from build123d import *

# Parameters (mm, degrees)
SKETCH1_R          = 10.5
EXTRUDE1_DEPTH     = 40
SKETCH2_R          = 2.5
EXTRUDE2_DEPTH     = 22.5
SKETCH3_R          = 13
SKETCH3_R_2        = 10.5
EXTRUDE3_DEPTH     = 3
SKETCH4_R          = 1.5
CUT_EXTRUDE1_DEPTH = 14
SKETCH7_R          = 2.2
CUT_EXTRUDE2_DEPTH = 1.5
CUT_EXTRUDE2_DRAFT = -26
SKETCH8_R          = 2.2
CUT_EXTRUDE3_DEPTH = 1.5
CUT_EXTRUDE3_TAPER = 26


with BuildPart() as part:
    # Sketch1 → Extrude1 (new body)
    with BuildSketch(Plane(origin=(0, 0, 0), x_dir=(1, 0, 0), z_dir=(0, 1, 0))):
        with Locations(Location((0, 0, 0), (0, 0, 270))):
            Circle(SKETCH1_R)
    extrude(amount=EXTRUDE1_DEPTH)

    # Sketch2 → Extrude2 (cut)
    with BuildSketch(Plane.XZ):
        with Locations(Location((0, 0, 0), (0, 0, 270))):
            Circle(SKETCH2_R)
    extrude(amount=-EXTRUDE2_DEPTH, mode=Mode.SUBTRACT)

    # Sketch3 → Extrude3 (add)
    with BuildSketch(Plane.XZ.offset(-6)):
        with Locations(Location((0, 0, 0), (0, 0, 270))):
            Circle(SKETCH3_R)
        with Locations(Location((0, 0, 0), (0, 0, 270))):
            Circle(SKETCH3_R_2, mode=Mode.SUBTRACT)
    extrude(amount=-EXTRUDE3_DEPTH)

    # Sketch4 → Cut-Extrude1 (cut, symmetric)
    with BuildSketch(Plane.XY):
        with Locations((0, 15.131749204)):
            Circle(SKETCH4_R)
    extrude(amount=CUT_EXTRUDE1_DEPTH, both=True, mode=Mode.SUBTRACT)


with BuildPart() as cut_extrude2_tool:
    # Sketch7 → Cut-Extrude2 (with draft: the straight prism first)
    with BuildSketch(Plane(origin=(0, 24.5, 10.5), x_dir=(-1, 0, 0), z_dir=(0, 0, 1))):
        with Locations((0, 9.368250796)):
            Circle(SKETCH7_R)
    extrude(amount=-CUT_EXTRUDE2_DEPTH)
    # Cut-Extrude2: the draft: its side faces are tilted about the plane it starts from
    cut_extrude2_sides = [cut_extrude2_tool.faces().sort_by_distance(p)[0] for p in [
        (2.2, 15.131749204, 9.75),
    ]]
    draft(cut_extrude2_sides, Plane(origin=(0, 24.5, 10.5), x_dir=(-1, 0, 0), z_dir=(0, 0, 1)), CUT_EXTRUDE2_DRAFT)


with BuildPart() as part_1:
    add(part.part)

    # Cut-Extrude2: cut by cut_extrude2_tool
    add(cut_extrude2_tool.part, mode=Mode.SUBTRACT)

    # Sketch8 → Cut-Extrude3 (cut)
    with BuildSketch(Plane.XY.offset(-10.5)):
        with Locations((0, 15.131749204)):
            Circle(SKETCH8_R)
    extrude(amount=CUT_EXTRUDE3_DEPTH, taper=CUT_EXTRUDE3_TAPER, mode=Mode.SUBTRACT)


solid = part_1.part
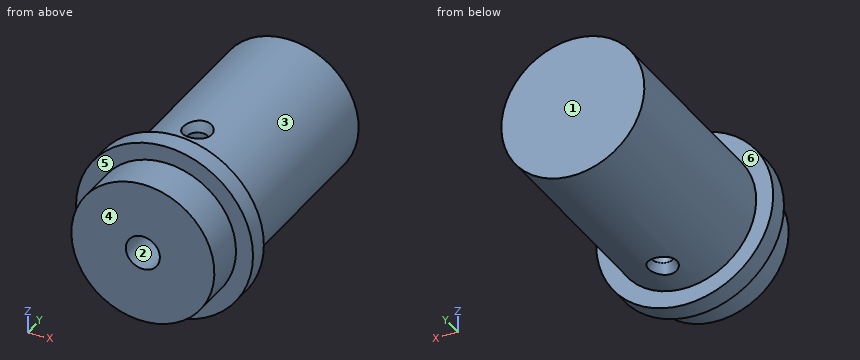
Read the model definition and answer for the solid it produces. Units are mm, in the model's axes. Face numbers are marked on the shaded views. A direction names the side the tool comes from. Round coordinates to 2 decimals unless told otherwise and drop trailing zeros. Order: outer loops, then holes, each group sorted by start corner. A loop starts at its lowest first (then second) coordinate and runs counter-clockwise, first axis right, second up.
1) The part is cut by section A-A on x = 0. Write down the section's boundary in (y, z), plus the area to 3 significant figures.
2) The part is cut by section C-C on z = 6.75. Write down the section's boundary in (x, y), plus the area to 3 significant figures.
3) The mould has two halves that part along X. Classify the marked faces 1, 2 and 3: released by +X, released by -X, zero draft, split by the parting line, or undercut.
4) For the marked faces 4, 5 and 6, determine the directions among +Z, -Z, +X, -X, +Y, -Y from which every point of the face is accessible in a straight line to the end or side of a thin tool.
5) Straight lines are drawn through the part: L1, parallel to Y at x = 0, z = 5.75; L2, parallel to Y at x = -1.5, z = -11.25; L3, parallel to Y at x = 0.25, z = -4.5. For each, find the intervals that lie inside material, in ascending order.
6) The part is cut by section D-D on x = 7.75. Write down the section's boundary in (y, z), plus the area to 3 significant figures.
7) Flat-ended cylindrical pins translate along their axes: pin 1 (3 mm diameter, centred on x = 1.5, y = 15.5, fed in from -Z); pin 2 (1 mm diameter, centred on y = 19, z = -0.5, fed in from +X); pin 3 (8 mm diameter, centred on y = 35, z = 1.5, fed in from -X); pin 4 (2.5 mm diameter, centred on x = 0, y = 15.13, fed in from +Z). Find the tip coordinate at first contact, or state that the pin passes through.
8) The part is cut by section B-B on z = 0. Write down the section's boundary in (x, y), plus the area to 4 significant figures.
Resolved:
1. outline: (0, -10.5) - (6, -10.5) - (6, -13) - (9, -13) - (9, -10.5) - (12.93, -10.5) - (13.63, -9.06) - (13.63, -2.5) - (0, -2.5) - close; (0, 2.5) - (13.63, 2.5) - (13.63, 9.06) - (12.93, 10.5) - (9, 10.5) - (9, 13) - (6, 13) - (6, 10.5) - (0, 10.5) - close; (16.63, -9.06) - (17.33, -10.5) - (40, -10.5) - (40, 10.5) - (17.33, 10.5) - (16.63, 9.06) - (16.63, 2.5) - (22.5, 2.5) - (22.5, -2.5) - (16.63, -2.5) - close
1. area: 692 mm2
2. outline: (-11.11, 6) - (-8.04, 6) - (-8.04, 0) - (8.04, 0) - (8.04, 6) - (11.11, 6) - (11.11, 9) - (8.04, 9) - (8.04, 40) - (-8.04, 40) - (-8.04, 9) - (-11.11, 9) - close; hole circle Ø3 at (0, 15.13)
2. area: 655 mm2
3. face 1: zero draft
3. face 2: undercut
3. face 3: split by the parting line
4. face 4: +Z, -Z, +X, -X, -Y
4. face 5: -Y
4. face 6: +Y
5. L1: y = 0 to 13.63, 16.63 to 40
5. L2: y = 6 to 9
5. L3: y = 0 to 13.65, 16.61 to 40
6. outline: (0, -7.08) - (6, -7.08) - (6, -10.44) - (9, -10.44) - (9, -7.08) - (40, -7.08) - (40, 7.08) - (9, 7.08) - (9, 10.44) - (6, 10.44) - (6, 7.08) - (0, 7.08) - close
6. area: 587 mm2
7. pin 1: stops at z = -10.44
7. pin 2: stops at x = 10.5
7. pin 3: stops at x = -10.5
7. pin 4: passes through
8. outline: (-13, 6) - (-10.5, 6) - (-10.5, 0) - (-2.5, 0) - (-2.5, 22.5) - (2.5, 22.5) - (2.5, 0) - (10.5, 0) - (10.5, 6) - (13, 6) - (13, 9) - (10.5, 9) - (10.5, 40) - (-10.5, 40) - (-10.5, 9) - (-13, 9) - close
8. area: 742.5 mm2
